The figure shows three views and two pictorial views of one solid part (mm, origin at its lowest corner). Answer the questions. Coordinates: 2 decimals unless noted, no trailing zeros. Order: outer loops, then holes, each group sorted by start corner. A loop starts at its lowest first (then second) coordinate and runs counter-clockwise, first axis right, second up. Notation, with made-up numbers: M 25.5,16 L 66.5,16 A28 cw 66.5,45 Z; hole C 51,-37.75 d5. An arc over 180 degrees is marked long. Use a Markdown table: item, result.
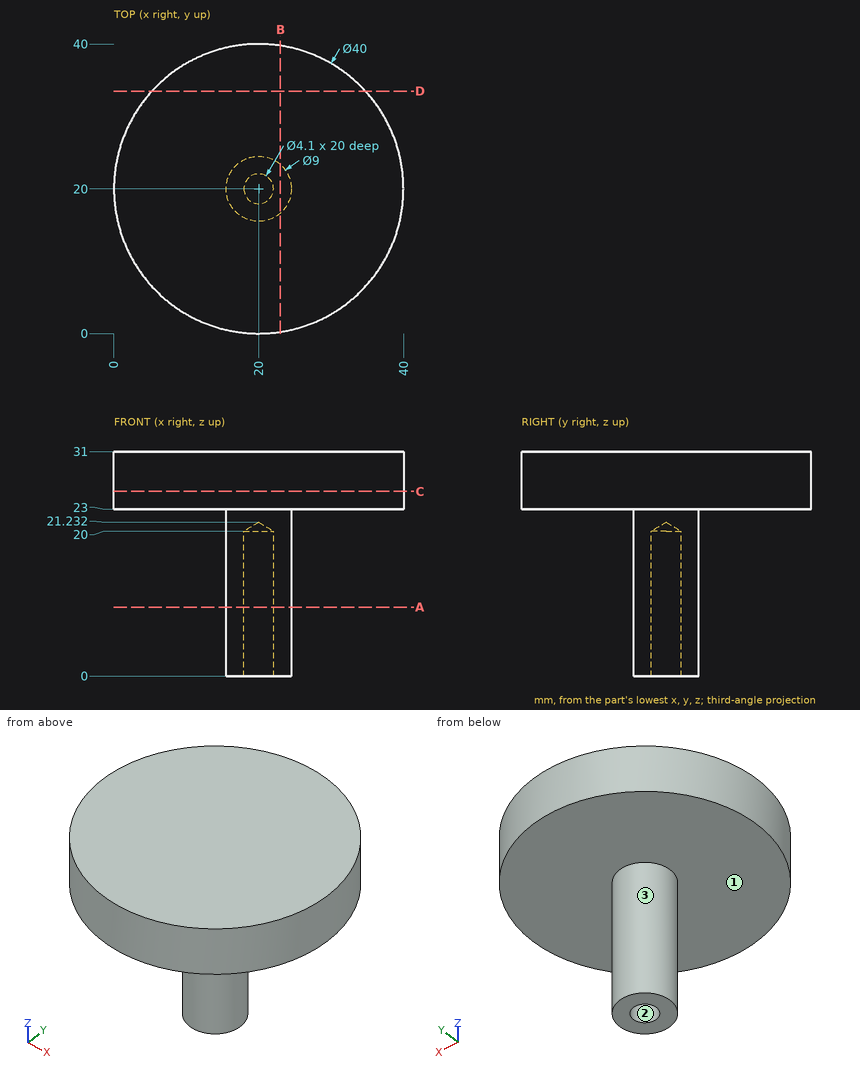
1. Section A-A on z = 9.5 is taken. Determine the outline of the cut face in (x, y), then the cut area to 3 significant figures.
Answers below:
| item | result |
|---|---|
| outline | C 20,20 d9; hole C 20,20 d4.1 |
| area | 50.4 mm² |
2. Section B-B on x = 23 is taken. Determine the outline of the cut face in (y, z).
Answers below:
| item | result |
|---|---|
| outline | M 0.23,23 L 16.65,23 L 16.65,0 L 23.35,0 L 23.35,23 L 39.77,23 L 39.77,31 L 0.23,31 Z |
3. Section C-C on z = 25.5 is taken. Determine the outline of the cut face in (x, y).
Answers below:
| item | result |
|---|---|
| outline | C 20,20 d40 |
4. Flat-ended cylindrical pins translate along their axes: P1, Ø12, axis at y = 7, z = 21.5, coming from the -X side; P2, Ø2, axis at x = 19.5, y = 35.5, coming from the -Z side. Find the tip coordinate at first contact, or state that the pin passes through.
Answers below:
| item | result |
|---|---|
| P1 | x = 1.34 |
| P2 | z = 23 |
5. Section D-D on y = 33.5 is taken. Determine the outline of the cut face in (x, z), then the cut area to 3 significant figures.
Answers below:
| item | result |
|---|---|
| outline | M 5.24,23 L 34.76,23 L 34.76,31 L 5.24,31 Z |
| area | 236 mm² |
6. Find the intervals of material crossed by probe 1 along Y at (x, z) = (20, 8.25); probe 2 along Z at (x, y) = (13, 3), in increasing order.
Answers below:
| item | result |
|---|---|
| probe 1 | 15.5 to 17.95, 22.05 to 24.5 |
| probe 2 | 23 to 31 |
7. For a pull along X with two mould halves and no side action, classify the marked faces 1, 2 and 3 as +X half, -X half, draft (parallel to the pull), parting line (faces both ways), or undercut.
Answers below:
| item | result |
|---|---|
| face 1 | draft |
| face 2 | undercut |
| face 3 | parting line |
